For this review, take the finished solid that the model builds, in its own axes (mm). A direction names the side the tool comes from. Round coordinates to 2 decimals unless told otherwise and drop trailing zeros. Order: outer loops, then holes, each group sorted by start corner. A loop starts at its lowest first (then second) coordinate and runs counter-clockwise, first axis right, second up. Notation, with made-up numbers: (48, 64) -> (70, 64) arc R30 cw to (70, 102) -> close; hole circle Ø9 at (85, 16.25). An arc over 180 degrees is marked (long way). Put each result on its own line as item: value. Start each with the question number.
```python
from build123d import *

# Parameters (mm, degrees)
SKETCH1_R             = 28.575
BOSS_EXTRUDE1_DEPTH   = 123.7
SKETCH2_R             = 26
BOSS_EXTRUDE2_DEPTH   = 81.3
SKETCH3_R             = 16
BOSS_EXTRUDE3_DEPTH   = 3
SKETCH4_R             = 6
BOSS_EXTRUDE4_DEPTH   = 22
CHAMFER1_SIZE         = 1
SKETCH6_R             = 3
CUT_EXTRUDE1_DEPTH    = 2
FILLET1_R             = 0.5
M5_TAPPED_HOLE1_D     = 4.2
M5_TAPPED_HOLE1_DEPTH = 12.4
M5_TAPPED_HOLE1_TIP   = 1.2618073
BOSS_EXTRUDE6_DEPTH   = 15
SKETCH14_R            = 1.75
BOSS_EXTRUDE7_DEPTH   = 5
CUT_EXTRUDE3_DEPTH    = 10


with BuildPart() as part:
    # Sketch1 → Boss-Extrude1 (new body)
    with BuildSketch(Plane(origin=(0, 0, 0), x_dir=(0, 0, -1), z_dir=(1, 0, 0))):
        Circle(SKETCH1_R)
    extrude(amount=BOSS_EXTRUDE1_DEPTH)

    # Sketch2 → Boss-Extrude2 (add)
    with BuildSketch(Plane(origin=(205, 0, 0), x_dir=(0, 0, -1), z_dir=(1, 0, 0))):
        Circle(SKETCH2_R)
    extrude(amount=-BOSS_EXTRUDE2_DEPTH)

    # Sketch3 → Boss-Extrude3 (add)
    with BuildSketch(Plane(origin=(205, 0, 0), x_dir=(0, 0, -1), z_dir=(1, 0, 0))):
        Circle(SKETCH3_R)
    extrude(amount=BOSS_EXTRUDE3_DEPTH)

    # Sketch4 → Boss-Extrude4 (add)
    with BuildSketch(Plane(origin=(208, 0, 0), x_dir=(0, 0, -1), z_dir=(1, 0, 0))):
        Circle(SKETCH4_R)
    extrude(amount=BOSS_EXTRUDE4_DEPTH)

    # Chamfer1
    chamfer1_edges = [part.edges().sort_by_distance(p)[0] for p in [
        (230, 0, 6),
    ]]
    chamfer(chamfer1_edges, length=CHAMFER1_SIZE)

    # Sketch6 → Cut-Extrude1 (cut)
    with BuildSketch(Plane(origin=(230, 0, 0), x_dir=(0, 0, -1), z_dir=(1, 0, 0))):
        Circle(SKETCH6_R)
    extrude(amount=-CUT_EXTRUDE1_DEPTH, mode=Mode.SUBTRACT)

    # Fillet1
    fillet1_edges = [part.edges().sort_by_distance(p)[0] for p in [
        (0, 0, 28.575),
        (123.7, 0, 28.575),
        (123.7, 0, 26),
        (205, 0, 26),
    ]]
    fillet(fillet1_edges, radius=FILLET1_R)

    # Sketch8 → M4 Tapped Hole1 (revolve, cut)
    with BuildSketch(Plane(origin=(230, 0, 0), x_dir=(0, 0, -1), z_dir=(0, 1, 0))):
        Polygon((0, 0), (0, 12.991420021), (1.65, 12), (1.65, 10), (2, 10), (2, 0), align=None)
    revolve(axis=Axis((236.35, 0, 0), (-1, 0, 0)), mode=Mode.SUBTRACT)

    # M5 Tapped Hole1
    with Locations(Plane(origin=(205, 14.142135624, -14.142135624), x_dir=(0, 0, 1), z_dir=(1, 0, 0))):
        with Locations((0, 0), (28.284271248, 0), (0, 28.284271248), (28.284271248, 28.284271248)):
            Hole(M5_TAPPED_HOLE1_D / 2, depth=M5_TAPPED_HOLE1_DEPTH)
            with Locations((0, 0, -(M5_TAPPED_HOLE1_DEPTH + M5_TAPPED_HOLE1_TIP / 2))):  # 118° drill point
                Cone(0, M5_TAPPED_HOLE1_D / 2, M5_TAPPED_HOLE1_TIP, mode=Mode.SUBTRACT)

    # Sketch13 → Boss-Extrude6 (add)
    with BuildSketch(Plane.ZY):
        with BuildLine():
            Line((-15, 18.575), (15, 18.575))
            Line((15, 18.575), (15, -4.425))
            ThreePointArc((15, -4.425), (0, -19.425), (-15, -4.425))
            Line((-15, -4.425), (-15, 18.575))
        make_face()
    extrude(amount=BOSS_EXTRUDE6_DEPTH)

    # Sketch14 → Boss-Extrude7 (add)
    # profile 1 of 2: a face of its own
    with BuildSketch(Plane.ZY):
        with BuildLine():
            Line((20, 4), (15, 6.331538291))
            Line((15, 6.331538291), (15, -6.331538291))
            Line((15, -6.331538291), (20, -4))
            ThreePointArc((20, -4), (24, 0), (20, 4))
        make_face()
        with Locations((20, 0)):
            Circle(SKETCH14_R, mode=Mode.SUBTRACT)
    # profile 2 of 2: a face of its own
    with BuildSketch(Plane.ZY):
        with BuildLine():
            Line((-20, -4), (-15, -6.331538291))
            Line((-15, -6.331538291), (-15, 6.331538291))
            Line((-15, 6.331538291), (-20, 4))
            ThreePointArc((-20, 4), (-24, 0), (-20, -4))
        make_face()
        with Locations(Location((-20, 0, 0), (0, 0, 180))):
            Circle(SKETCH14_R, mode=Mode.SUBTRACT)
    extrude(amount=BOSS_EXTRUDE7_DEPTH)

    # Sketch15 → Cut-Extrude3 (cut)
    with BuildSketch(Plane(origin=(0, 4, 0), x_dir=(1, 0, 0), z_dir=(0, 1, 0))):
        with BuildLine():
            Line((225, -2), (213, -2))
            ThreePointArc((213, -2), (211, 0), (213, 2))
            Line((213, 2), (225, 2))
            ThreePointArc((225, 2), (227, 0), (225, -2))
        make_face()
    extrude(amount=CUT_EXTRUDE3_DEPTH, mode=Mode.SUBTRACT)


solid = part.part
```
Item 1: For L1, parallel to Y at x = -2.75, z = -20; L2, parallel to Y at x = 222, z = 0; L3, parallel to Y at x = 195.5, z = 20.5, list the stretches that pass through material, from the lowest coordinate up.
Item 2: Consider section B-B, the plane x = 171.5. Write out the cut boundary in (y, z), plus the area to 3 significant figures.
Item 3: Insertion check: pin 1 Ø6.5 at (y, z) = (14.14, -14.14) entering from +X; pin 2 Ø12 at (x, y) = (149, 21) entering from -Z; pin 3 Ø2 at (x, y) = (68.5, -11) entering from +Z. Each pin has a flat end and moves straight along its axis. Give the tip position at first contact, or say it passes through.
Item 4: Tool access review of faces 1 (the face through (-2.465, -5.149, -17.535)), 2 (the face through (-9, 7, -15)), 3 (the face through (-5, 0, 17)), 4 (the face through (-2, 0, 24)), 5 (the face through (206.48, -15.62, 3.47)): name each direction out of +Z, -Z, +X, -X, +Y, -Y from which nothing blocks a thin tool from reaching the whole face with its end or side.
Item 5: Mouldability with a two-part tool opening along Y and no side actions: class faces 6 (the face through (-2.465, -5.182, 17.465)), 7 (the face through (198.713, 15.42, -12.476)), 8 (the face through (205, 12, -11)) as +Y half, -Y half, draft (parallel to the pull), parting line (faces both ways), or undercut.
Item 6: Consider section A-A, the plane x = 57.5. Write out the cut boundary in (y, z) (3 decimals).
Evaluation:
1. L1: y = -4 to -1.75, 1.75 to 4
1. L2: y = -6 to -2, 2 to 4
1. L3: y = -15.99 to 15.99
2. outline: circle Ø52 at (0, 0)
2. area: 2,120 mm^2
3. pin 1: stops at x = 205
3. pin 2: stops at z = -21.24
3. pin 3: stops at z = 26.77
4. face 1: -Z, -X, -Y
4. face 2: -Z, -X, +Y
4. face 3: +Z, -X, +Y, -Y
4. face 4: +Z, -X
4. face 5: +X
5. face 6: -Y half
5. face 7: undercut
5. face 8: draft
6. outline: circle Ø57.15 at (0, 0)
